Geometry check sheet. Reference: the model listing, model coordinates, mm. Round coordinates to 2 decimals unless told otherwise and drop trailing zeros. Loops run counter-clockwise (first coordinate to the right, second up) from the corner with the lowest first, then second, coordinate; pieces in that order, holes last.
```python
from build123d import *

# Parameters (mm, degrees)
SKETCH_1_W      = 75
SKETCH_1_H      = 45
SKETCH_1_R      = 12.1
SKETCH_1_R_2    = 2.15
EXTRUDE_1_DEPTH = 3
FILLET_1_R      = 10


with BuildPart() as part:
    # ｽｹｯﾁ1 → ﾎﾞｽ - 押し出し1 (new body)
    with BuildSketch(Plane.XY):
        with Locations((37.5, 22.5)):
            Rectangle(SKETCH_1_W, SKETCH_1_H)
        with Locations((19.5, 25)):
            Circle(SKETCH_1_R, mode=Mode.SUBTRACT)
        with Locations((55.5, 25)):
            Circle(SKETCH_1_R, mode=Mode.SUBTRACT)
        with Locations((5, 5)):
            Circle(SKETCH_1_R_2, mode=Mode.SUBTRACT)
        with Locations(Location((70, 5, 0), (0, 0, 180))):
            Circle(SKETCH_1_R_2, mode=Mode.SUBTRACT)
    extrude(amount=EXTRUDE_1_DEPTH)

    # ﾌｨﾚｯﾄ1
    fillet_1_edges = [part.edges().sort_by_distance(p)[0] for p in [
        (0, 45, 1.5),
        (75, 45, 1.5),
    ]]
    fillet(fillet_1_edges, radius=FILLET_1_R)


solid = part.part
```
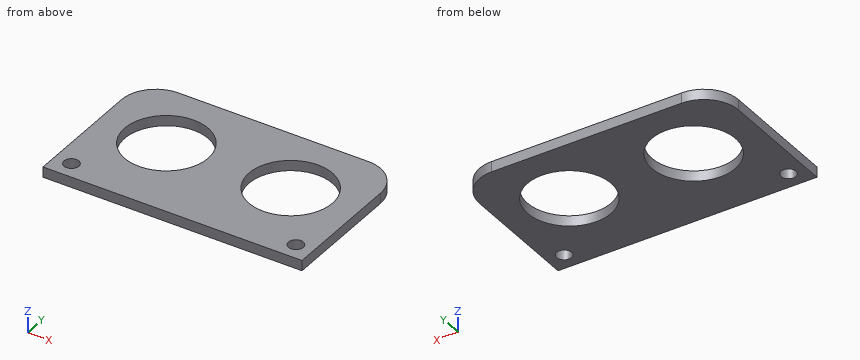
1) Sectioned sample at C-C, the plane z = 0.6. Record the cut outline in (x, y).
Report:
outline: (0, 0) - (75, 0) - (75, 35) arc R10 ccw to (65, 45) - (10, 45) arc R10 ccw to (0, 35) - close; hole circle Ø4.3 at (5, 5); hole circle Ø24.2 at (19.5, 25); hole circle Ø24.2 at (55.5, 25); hole circle Ø4.3 at (70, 5)
2) Scan lines: line 1 along Y through (x, z) = (19.5, 2.2); line 2 along X through (y, z) = (35.5, 2); line 3 along X through (y, z) = (20.5, 2.45). Record each from-to range of solid material in increasing order.
Report:
line 1: y = 0 to 12.9, 37.1 to 45
line 2: x = 0.01 to 13.49, 25.51 to 49.49, 61.51 to 74.99
line 3: x = 0 to 8.27, 30.73 to 44.27, 66.73 to 75
3) Sectioned sample at D-D, the plane y = 33. Record the cut outline in (x, z).
Report:
outline: (0, 0) - (10.42, 0) - (10.42, 3) - (0, 3) - close; (28.58, 0) - (46.42, 0) - (46.42, 3) - (28.58, 3) - close; (64.58, 0) - (75, 0) - (75, 3) - (64.58, 3) - close
4) Gauge pin test, flat end, axial feed: pin 1 (22 mm diameter, centred on x = 55.5, y = 25, fed in from +Z). Record the tip position at first contact, or that the pin passes through.
Report:
pin 1: passes through
5) Sectioned sample at B-B, the plane x = 55.5. Record the cut outline in (y, z), then the cut area to 3 significant figures.
Report:
outline: (0, 0) - (12.9, 0) - (12.9, 3) - (0, 3) - close; (37.1, 0) - (45, 0) - (45, 3) - (37.1, 3) - close
area: 62.4 mm2
6) Sectioned sample at A-A, the plane y = 5. Record the cut outline in (x, z), then the cut area to 3 significant figures.
Report:
outline: (0, 0) - (2.85, 0) - (2.85, 3) - (0, 3) - close; (7.15, 0) - (67.85, 0) - (67.85, 3) - (7.15, 3) - close; (72.15, 0) - (75, 0) - (75, 3) - (72.15, 3) - close
area: 199 mm2
